```python
from build123d import *

# Parameters (mm, degrees)
F0_R     = 6
F0_R_2   = 2.5
F0_W     = 79
F0_H     = 52
F1_DEPTH = 85
F2_DEPTH = 77
F3_W     = 8
F3_H     = 52
F4_DEPTH = 81.5
F6_DEPTH = 150


with BuildPart() as f1:
    # F0 (on Top) → F1 (new body)
    with BuildSketch(Plane.XY):
        with BuildLine():
            Line((0, 95), (0, 0))
            Line((0, 0), (150, 0))
            Line((150, 0), (150, 95))
            ThreePointArc((150, 95), (148.535534, 98.535534), (145, 100))
            Line((145, 100), (5, 100))
            ThreePointArc((5, 100), (1.464466, 98.535534), (0, 95))
        make_face()
        Polygon((140, 94), (140, 18), (49, 18), (10, 18), (10, 94.470508), (49, 94), align=None, mode=Mode.SUBTRACT)
        Polygon((49, 18), (140, 18), (140, 94), (49, 94), (10, 94.470508), (10, 18), align=None)
        with Locations((24.5, 42.768653)):
            Circle(F0_R, mode=Mode.SUBTRACT)
        with Locations((24.5, 56)):
            Circle(F0_R_2, mode=Mode.SUBTRACT)
        with Locations((24.5, 69.2)):
            Circle(F0_R_2, mode=Mode.SUBTRACT)
        with Locations((88.5, 56)):
            Rectangle(F0_W, F0_H, mode=Mode.SUBTRACT)
    extrude(amount=F1_DEPTH)

    # F0 (on Top) → F2 (cut)
    with BuildSketch(Plane.XY):
        Polygon((49, 18), (140, 18), (140, 94), (49, 94), (10, 94.470508), (10, 18), align=None)
        with Locations((24.5, 42.768653)):
            Circle(F0_R, mode=Mode.SUBTRACT)
        with Locations((24.5, 56)):
            Circle(F0_R_2, mode=Mode.SUBTRACT)
        with Locations((24.5, 69.2)):
            Circle(F0_R_2, mode=Mode.SUBTRACT)
        with Locations((88.5, 56)):
            Rectangle(F0_W, F0_H, mode=Mode.SUBTRACT)
    extrude(amount=F2_DEPTH, mode=Mode.SUBTRACT)

    # F3 (on face) → F4 (cut)
    with BuildSketch(Plane.XY):
        with Locations((45, 56)):
            Rectangle(F3_W, F3_H)
    extrude(amount=F4_DEPTH, mode=Mode.SUBTRACT)

    # F5 (on face) → F6 (cut, through all)
    with BuildSketch(Plane(origin=(0, 0, 0), x_dir=(0, -1, 0), z_dir=(-1, 0, 0))):
        Polygon((0, 0), (0, 85), (-7.192497, 0), align=None)
    extrude(amount=-F6_DEPTH, mode=Mode.SUBTRACT)


solid = f1.part
```
Read the model definition and answer for the solid it produces. Units are mm, in the model's axes. A direction names the side the tool comes from. Give positions to 0.01 mm unless a question says otherwise; leave off trailing zeros. Order: outer loops, then holes, each group sorted by start corner. A loop starts at its lowest first (then second) coordinate and runs counter-clockwise, first axis right, second up.
(1) Find section C-C (x = 114). Give the vertices of the cut face in (y, z), plus the area to 3 significant figures.
(2) Find section B-B (y = 32). Give the vertices of the cut face in (x, z), plus the area to 3 significant figures.
(3) Find section A-A (y = 56). Give the vertices of the cut face in (x, z), plus the area to 3 significant figures.
(4) Given pin 1 (2.5 mm diameter, centred on x = 82, z = 82, fed in from -Y); pin 2 (6 mm diameter, centred on x = 24.5, y = 69.2, fed in from -Z); pin 3 (1.5 mm diameter, centred on x = 69, z = 12.5, fed in from -Y), each flat-ended and moving along its own axis, determine where each tip first touches the part or whether it passes through.
(5) For faces 1 (the flat face through (73.95, 3.546, 43.095)), 2 (the flat face through (95, 94, 38)), determine the directions among +Z, -Z, +X, -X, +Y, -Y from which every point of the face is accessible in a straight line to the end or side of a thin tool.
(6) Straight lines are drawn through the part: L1, parallel to X at y = 69, z = 79; L2, parallel to X at y = 20, z = 52; L3, parallel to Y at x = 24.5, z = 80.5. For each, find the intervals that lie inside material, in ascending order.
(7) For a pull along Y with two mould halves and no side action, classify faces 3 (the flat face through (74, 13, 0)), 4 (the flat face through (128, 56, 81)), 5 (the flat face through (49, 56, 83)), 6 (the cylindrical face through (149, 98, 42)) as released by +Y, released by -Y, zero draft, split by the parting line, or undercut.
(8) Find section D-D (z = 21). Give the vertices of the cut face in (x, y), plus the area to 3 significant figures.
Result sheet:
1. outline: (0, 85) - (7.19, 0) - (18, 0) - (18, 77) - (30, 77) - (30, 85) - close; (82, 77) - (94, 77) - (94, 0) - (100, 0) - (100, 85) - (82, 85) - close
1. area: 1,930 mm2
2. outline: (0, 0) - (10, 0) - (10, 77) - (41, 77) - (41, 81.5) - (49, 81.5) - (49, 85) - (0, 85) - close; (128, 77) - (140, 77) - (140, 0) - (150, 0) - (150, 85) - (128, 85) - close
2. area: 2,070 mm2
3. outline: (0, 0) - (10, 0) - (10, 77) - (22, 77) - (22, 85) - (0, 85) - close; (27, 77) - (41, 77) - (41, 81.5) - (49, 81.5) - (49, 85) - (27, 85) - close; (128, 77) - (140, 77) - (140, 0) - (150, 0) - (150, 85) - (128, 85) - close
3. area: 2,030 mm2
4. pin 1: stops at y = 0.15
4. pin 2: stops at z = 77
4. pin 3: stops at y = 6.07
5. face 1: -Z, +X, -X, -Y
5. face 2: -Z
6. L1: x = 0 to 22.01, 26.99 to 41, 128 to 150
6. L2: x = 0 to 10, 140 to 150
6. L3: y = 0.38 to 36.77, 48.77 to 53.5, 58.5 to 66.7, 71.7 to 100
7. face 3: zero draft
7. face 4: undercut
7. face 5: undercut
7. face 6: released by +Y
8. outline: (0, 5.42) - (150, 5.42) - (150, 95) arc R5 ccw to (145, 100) - (5, 100) arc R5 ccw to (0, 95) - close; hole (10, 18) - (140, 18) - (140, 94) - (49, 94) - (10, 94.47) - close
8. area: 4,290 mm2
